```python
from build123d import *

# Parameters (mm, degrees)
SKETCH1_R           = 7.5
BOSS_EXTRUDE1_DEPTH = 18
SKETCH2_W           = 399.543241252
SKETCH2_H           = 23.51775922
BOSS_EXTRUDE2_DEPTH = 7


with BuildPart() as part:
    # Sketch1 → Boss-Extrude1 (new body)
    with BuildSketch(Plane(origin=(0, 0, 0), x_dir=(0, 0, -1), z_dir=(1, 0, 0))):
        Circle(SKETCH1_R)
    extrude(amount=BOSS_EXTRUDE1_DEPTH)

    # Sketch2 → Boss-Extrude2 (add)
    with BuildSketch(Plane(origin=(18, 0, 0), x_dir=(0, 0, -1), z_dir=(1, 0, 0))):
        with Locations((-186.816113962, 0)):
            Rectangle(SKETCH2_W, SKETCH2_H)
    extrude(amount=BOSS_EXTRUDE2_DEPTH)


solid = part.part
```
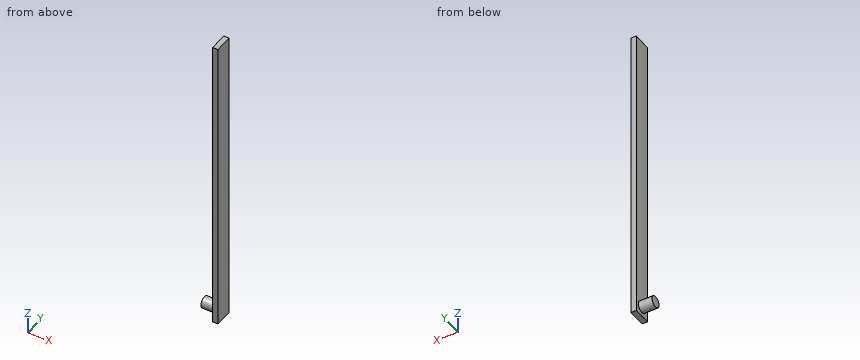
CAD build for the part. Positions are in the model's coordinates, mm. Coordinates: 2 decimals unless noted, no trailing zeros. Order: outer loops, then holes, each group sorted by start corner. A loop starts at its lowest first (then second) coordinate and runs counter-clockwise, first axis right, second up. Notation, with made-up numbers: M 69.25,-30.75 L 94.25,-30.75 A15 cw 94.25,-13.75 Z; hole C -28,-12.75 d8. An arc over 180 degrees is marked long. Write each question's results on one line, items separated by ' | '. Start each with the question number.
Q1. Drill centre lines: probe 1 along X at (y, z) = (6.25, 51.5); probe 2 along Z at (x, y) = (13.5, 5); probe 3 along Z at (x, y) = (5.5, 2.5). Where is each one in solid material? Low to high. Write a range as from..to.
Q2. Cut at C-C (x = 8). List the corners of the cut face in (y, z).
Q3. Cut at B-B (z = 0). List the corners of the cut face in (x, y), then the cut area to 3 significant figures.
Q4. Cut at A-A (y = 3.25). List the corners of the cut face in (x, z), then the cut area to 3 significant figures.
Q5. Cut at D-D (z = 199). List the corners of the cut face in (x, y), then the cut area to 3 significant figures.
Q6. Flat gauge pins, fed straight in: P1, Ø6, axis at x = 4, y = 0, coming from the +Z side; P2, Ø12, axis at x = 17, y = 3, coming from the -Z side; P3, Ø7, axis at y = -4, z = 143.5, coming from the -X side; P4, Ø12, axis at x = 6.5, y = -7, coming from the -Z side. Where does each tip first touch, or does it go through?
Found:
1) probe 1: 18..25 | probe 2: -5.59..5.59 | probe 3: -7.07..7.07
2) outline: C 0,0 d15
3) outline: M 0,-7.5 L 18,-7.5 L 18,-11.76 L 25,-11.76 L 25,11.76 L 18,11.76 L 18,7.5 L 0,7.5 Z | area: 435 mm²
4) outline: M 0,-6.76 L 18,-6.76 L 18,-12.96 L 25,-12.96 L 25,386.59 L 18,386.59 L 18,6.76 L 0,6.76 Z | area: 3,040 mm²
5) outline: M 18,-11.76 L 25,-11.76 L 25,11.76 L 18,11.76 Z | area: 165 mm²
6) P1: z = 7.5 | P2: z = -12.96 | P3: x = 18 | P4: z = -7.43
